Source: CAD feature listing. Evaluate the final solid. Frame: model axes, mm. Face numbers are marked on the shaded views. A direction names the side the tool comes from. Round coordinates to 2 decimals unless told otherwise and drop trailing zeros. Loops run counter-clockwise (first coordinate to the right, second up) from the corner with the lowest first, then second, coordinate; pieces in that order, holes last.
Item 1: Section query D-D on z = 10.25. Return loops of the section in (x, y), then the cut area to 3 significant figures.
Item 2: Section query A-A on z = 21.75. Return loops of the section in (x, y), then the cut area to 3 significant figures.
Item 3: Section query B-B on y = 0. Return loops of the section in (x, z), then the cut area to 3 significant figures.
Item 4: First-contact query: P1, Ø4, axis at x = 4.5, y = 4, coming from the -Z side; P2, Ø1.5, axis at y = -4.5, z = 10.5, coming from the -X side; P3, Ø5, axis at y = 0, z = 20.5, coming from the +X side; P4, Ø7, axis at x = 1, z = 19, coming from the -Y side. Flat tips, straight axial feed; report the tip coordinate or a pass-through.
Item 5: Ray query, L1, parallel to Z at x = -1.5, y = 4.25; L2, parallel to Y at x = 1.5, z = 19.5; L3, parallel to Y at x = -0.5, z = 16. Return the intervals inside material, ascending.
Item 6: Access query for the marked faces 1 and 2. Directions: +Z, -Z, +X, -X, +Y, -Y. A direction counts if a zero-diameter tool reaches every point of the face in a straight line with its end or side. Return the directions, or none.
Item 7: Section query C-C on x = 0. Return loops of the section in (y, z), then the cut area to 3 significant figures.
```python
from build123d import *

# Parameters (mm, degrees)
F0_R     = 3.35
F1_DEPTH = 25
F0_R_2   = 6
F2_DEPTH = 5
F4_DEPTH = 10


with BuildPart() as f1:
    # F0 (on Top) → F1 (new body)
    with BuildSketch(Plane.XY):
        Circle(F0_R)
    extrude(amount=F1_DEPTH)

    # F0 (on Top) → F2 (join)
    with BuildSketch(Plane.XY):
        Circle(F0_R_2)
        Circle(F0_R, mode=Mode.SUBTRACT)
    extrude(amount=F2_DEPTH)

    # F3 (on face) → F4 (cut)
    with BuildSketch(Plane.XY.offset(25)):
        with BuildLine():
            ThreePointArc((-3.1972644557, 1), (-3.35, 0), (-3.1972644557, -1))
            Line((-3.1972644557, -1), (3.1972644557, -1))
            ThreePointArc((3.1972644557, -1), (3.3115959843, -0.505798415), (3.35, 0))
            ThreePointArc((3.35, 0), (3.3115959843, 0.505798415), (3.1972644557, 1))
            Line((3.1972644557, 1), (-3.1972644557, 1))
        make_face()
    extrude(amount=-F4_DEPTH, mode=Mode.SUBTRACT)


solid = f1.part
```
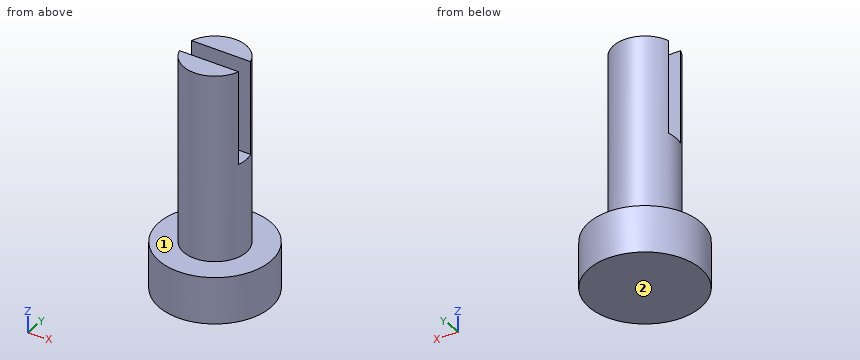
Data:
1. outline: circle Ø6.7 at (0, 0)
1. area: 35.3 mm2
2. outline: (-3.2, -1) arc R3.35 ccw to (3.2, -1) - close; (-3.2, 1) - (3.2, 1) arc R3.35 ccw to start
2. area: 22.1 mm2
3. outline: (-6, 0) - (6, 0) - (6, 5) - (3.35, 5) - (3.35, 15) - (-3.35, 15) - (-3.35, 5) - (-6, 5) - close
3. area: 127 mm2
4. P1: stops at z = 0
4. P2: passes through
4. P3: stops at x = 3.2
4. P4: stops at y = -3.35
5. L1: z = 0 to 5
5. L2: y = -3 to -1, 1 to 3
5. L3: y = -3.31 to -1, 1 to 3.31
6. face 1: +Z
6. face 2: -Z, +X, -X, +Y, -Y
7. outline: (-6, 0) - (6, 0) - (6, 5) - (3.35, 5) - (3.35, 25) - (1, 25) - (1, 15) - (-1, 15) - (-1, 25) - (-3.35, 25) - (-3.35, 5) - (-6, 5) - close
7. area: 174 mm2
